from build123d import *

# Parameters (mm, degrees)
SKETCH1_W            = 350
SKETCH1_H            = 340
BOSS_EXTRUDE1_DEPTH  = 6
CUT_EXTRUDE2_DEPTH   = 6
MIRROR2_COPY_1_DEPTH = 6
CUT_EXTRUDE3_DEPTH   = 6
SKETCH4_W            = 10
SKETCH4_H            = 82.256980738
CUT_EXTRUDE4_DEPTH   = 6
SKETCH5_R            = 2.25
SKETCH5_R_2          = 1.75
CUT_EXTRUDE5_DEPTH   = 6
SKETCH6_W            = 12
SKETCH6_H            = 9
CUT_EXTRUDE6_DEPTH   = 6
SKETCH8_W            = 5
SKETCH8_H            = 3
CUT_EXTRUDE7_DEPTH   = 6
LPATTERN1_COUNT      = 3
LPATTERN1_PITCH      = 50
SKETCH9_W            = 3
SKETCH9_H            = 5
CUT_EXTRUDE8_DEPTH   = 6
LPATTERN2_COUNT      = 4
LPATTERN2_PITCH      = 50
SKETCH10_W           = 30
SKETCH10_H           = 25
CUT_EXTRUDE9_DEPTH   = 6
SKETCH11_W           = 10
SKETCH11_H           = 51.49656536
CUT_EXTRUDE10_DEPTH  = 6
SKETCH12_W           = 45
SKETCH12_H           = 45
CUT_EXTRUDE11_DEPTH  = 6
FILLET2_R            = 4.9
SKETCH13_R           = 2.75
CUT_EXTRUDE12_DEPTH  = 6
SKETCH14_W           = 50
SKETCH14_H           = 20
SKETCH14_W_2         = 40
CUT_EXTRUDE13_DEPTH  = 10
FILLET4_R            = 5
FILLET5_R            = 5
SKETCH15_W           = 65
SKETCH15_H           = 46.515736948
CUT_EXTRUDE14_DEPTH  = 10
FILLET6_R            = 10


with BuildPart() as part:
    # Sketch1 → Boss-Extrude1 (new body)
    with BuildSketch(Plane(origin=(0, 0, 0), x_dir=(1, 0, 0), z_dir=(0, 1, 0))):
        Rectangle(SKETCH1_W, SKETCH1_H)
    extrude(amount=BOSS_EXTRUDE1_DEPTH)

    # Sketch2 → Cut-Extrude2 (cut)
    with BuildSketch(Plane(origin=(0, 6, 0), x_dir=(1, 0, 0), z_dir=(0, 1, 0))):
        Polygon((-175, -130), (-155, -130), (-155, -150), (-135, -150), (-135, -170), (-175, -170), align=None)
    cut_extrude2 = extrude(amount=-CUT_EXTRUDE2_DEPTH, mode=Mode.SUBTRACT)

    # Mirror1: Cut-Extrude2 across plane
    add(cut_extrude2.mirror(Plane.XY), mode=Mode.SUBTRACT)

    # Mirror2: Cut-Extrude2 across plane
    add(cut_extrude2.mirror(Plane(origin=(0, 0, 0), x_dir=(0, 0, 1), z_dir=(1, 0, 0))), mode=Mode.SUBTRACT)

    # Mirror2 copy 1 sketch → Mirror2 copy 1 (cut)
    with BuildSketch(Plane(origin=(0, 6, 0), x_dir=(-1, 0, 0), z_dir=(0, 1, 0))):
        Polygon((-175, -130), (-155, -130), (-155, -150), (-135, -150), (-135, -170), (-175, -170), align=None)
    extrude(amount=-MIRROR2_COPY_1_DEPTH, mode=Mode.SUBTRACT)

    # Sketch3 → Cut-Extrude3 (cut)
    with BuildSketch(Plane(origin=(0, 6, 0), x_dir=(1, 0, 0), z_dir=(0, 1, 0))):
        Polygon((-22.5, 170), (-22.5, 150), (-11.5, 112), (11.5, 112), (22.5, 150), (22.5, 170), align=None)
    extrude(amount=-CUT_EXTRUDE3_DEPTH, mode=Mode.SUBTRACT)

    # Sketch4 → Cut-Extrude4 (cut)
    with BuildSketch(Plane(origin=(0, 6, 0), x_dir=(1, 0, 0), z_dir=(0, 1, 0))):
        with Locations((-97.5, 165.128490369)):
            Rectangle(SKETCH4_W, SKETCH4_H)
        with Locations((97.5, 165.128490369)):
            Rectangle(SKETCH4_W, SKETCH4_H)
    extrude(amount=-CUT_EXTRUDE4_DEPTH, mode=Mode.SUBTRACT)

    # Sketch5 → Cut-Extrude5 (cut)
    with BuildSketch(Plane(origin=(0, 6, 0), x_dir=(1, 0, 0), z_dir=(0, 1, 0))):
        with Locations(Location((104, 51.5, 0), (0, 0, 270))):
            Circle(SKETCH5_R)
        with Locations(Location((104, -99, 0), (0, 0, 270))):
            Circle(SKETCH5_R)
        with Locations(Location((54, -99, 0), (0, 0, 270))):
            Circle(SKETCH5_R)
        with Locations(Location((54, 51.5, 0), (0, 0, 270))):
            Circle(SKETCH5_R)
        with Locations(Location((-4.5, 33.75, 0), (0, 0, 270))):
            Circle(SKETCH5_R_2)
        with Locations(Location((-4.5, -81.25, 0), (0, 0, 270))):
            Circle(SKETCH5_R_2)
        with Locations(Location((-96.5, -81.25, 0), (0, 0, 270))):
            Circle(SKETCH5_R_2)
        with Locations(Location((-96.5, 33.75, 0), (0, 0, 270))):
            Circle(SKETCH5_R_2)
    extrude(amount=-CUT_EXTRUDE5_DEPTH, mode=Mode.SUBTRACT)

    # Sketch6 → Cut-Extrude6 (cut)
    with BuildSketch(Plane(origin=(0, 6, 0), x_dir=(1, 0, 0), z_dir=(0, 1, 0))):
        with Locations((-97.5, 145.5)):
            Rectangle(SKETCH6_W, SKETCH6_H)
        with Locations((97.5, 145.5)):
            Rectangle(SKETCH6_W, SKETCH6_H)
    extrude(amount=-CUT_EXTRUDE6_DEPTH, mode=Mode.SUBTRACT)

    # Sketch8 → Cut-Extrude7 (cut)
    with BuildSketch(Plane(origin=(0, 6, 0), x_dir=(1, 0, 0), z_dir=(0, 1, 0))):
        with Locations((-4.5, -125)):
            Rectangle(SKETCH8_W, SKETCH8_H)
        with Locations((-4.5, -145)):
            Rectangle(SKETCH8_W, SKETCH8_H)
    cut_extrude7 = extrude(amount=-CUT_EXTRUDE7_DEPTH, mode=Mode.SUBTRACT)

    # LPattern1: Cut-Extrude7 ×3
    with Locations(*[(-i * LPATTERN1_PITCH, 0, 0) for i in range(1, LPATTERN1_COUNT)]):
        add(cut_extrude7, mode=Mode.SUBTRACT)

    # Sketch9 → Cut-Extrude8 (cut)
    with BuildSketch(Plane(origin=(0, 6, 0), x_dir=(1, 0, 0), z_dir=(0, 1, 0))):
        with Locations((-150, -81.25)):
            Rectangle(SKETCH9_W, SKETCH9_H)
        with Locations((-130, -81.25)):
            Rectangle(SKETCH9_W, SKETCH9_H)
    cut_extrude8 = extrude(amount=-CUT_EXTRUDE8_DEPTH, mode=Mode.SUBTRACT)

    # LPattern2: Cut-Extrude8 ×4
    with Locations(*[(0, 0, -i * LPATTERN2_PITCH) for i in range(1, LPATTERN2_COUNT)]):
        add(cut_extrude8, mode=Mode.SUBTRACT)

    # Sketch10 → Cut-Extrude9 (cut)
    with BuildSketch(Plane(origin=(0, 6, 0), x_dir=(1, 0, 0), z_dir=(0, 1, 0))):
        with Locations((140, -157.5)):
            Rectangle(SKETCH10_W, SKETCH10_H)
    cut_extrude9 = extrude(amount=-CUT_EXTRUDE9_DEPTH, mode=Mode.SUBTRACT)

    # Mirror3: Cut-Extrude9 across plane
    add(cut_extrude9.mirror(Plane(origin=(0, 0, 0), x_dir=(0, 0, 1), z_dir=(1, 0, 0))), mode=Mode.SUBTRACT)

    # Sketch11 → Cut-Extrude10 (cut)
    with BuildSketch(Plane(origin=(0, 6, 0), x_dir=(1, 0, 0), z_dir=(0, 1, 0))):
        with Locations((55, 165.74828268)):
            Rectangle(SKETCH11_W, SKETCH11_H)
    extrude(amount=-CUT_EXTRUDE10_DEPTH, mode=Mode.SUBTRACT)

    # Sketch12 → Cut-Extrude11 (cut)
    with BuildSketch(Plane(origin=(0, 6, 0), x_dir=(1, 0, 0), z_dir=(0, 1, 0))):
        with Locations((-152.5, 147.5)):
            Rectangle(SKETCH12_W, SKETCH12_H)
    extrude(amount=-CUT_EXTRUDE11_DEPTH, mode=Mode.SUBTRACT)

    # Fillet2
    fillet2_edges = [part.edges().sort_by_distance(p)[0] for p in [
        (125, 3, 145),
        (-125, 3, 145),
        (50, 3, -140),
        (60, 3, -140),
        (-130, 3, -125),
    ]]
    fillet(fillet2_edges, radius=FILLET2_R)

    # Sketch13 → Cut-Extrude12 (cut)
    with BuildSketch(Plane(origin=(0, 6, 0), x_dir=(1, 0, 0), z_dir=(0, 1, 0))):
        with Locations(Location((165, -120, 0), (0, 0, 270))):
            Circle(SKETCH13_R)
        with Locations(Location((165, 120, 0), (0, 0, 270))):
            Circle(SKETCH13_R)
        with Locations(Location((125, 160, 0), (0, 0, 270))):
            Circle(SKETCH13_R)
        with Locations(Location((-120, 160, 0), (0, 0, 270))):
            Circle(SKETCH13_R)
        with Locations(Location((-165, 115, 0), (0, 0, 270))):
            Circle(SKETCH13_R)
        with Locations(Location((-165, -120, 0), (0, 0, 270))):
            Circle(SKETCH13_R)
        with Locations(Location((-115, -160, 0), (0, 0, 270))):
            Circle(SKETCH13_R)
        with Locations(Location((115, -160, 0), (0, 0, 270))):
            Circle(SKETCH13_R)
    extrude(amount=-CUT_EXTRUDE12_DEPTH, mode=Mode.SUBTRACT)

    # Sketch14 → Cut-Extrude13 (cut)
    with BuildSketch(Plane(origin=(0, 6, 0), x_dir=(1, 0, 0), z_dir=(0, 1, 0))):
        with Locations((82.5, 160)):
            Rectangle(SKETCH14_W, SKETCH14_H)
        with Locations((-87.5, 160)):
            Rectangle(SKETCH14_W_2, SKETCH14_H)
    extrude(amount=-CUT_EXTRUDE13_DEPTH, mode=Mode.SUBTRACT)

    # Fillet4
    fillet4_edges = [part.edges().sort_by_distance(p)[0] for p in [
        (-102.5, 3, -124),
        (-92.5, 3, -124),
    ]]
    fillet(fillet4_edges, radius=FILLET4_R - 0.0001)  # a hair under: the kernel refuses the full size

    # Fillet5
    fillet5_edges = [part.edges().sort_by_distance(p)[0] for p in [
        (92.5, 3, -124),
        (102.5, 3, -124),
    ]]
    fillet(fillet5_edges, radius=FILLET5_R - 0.0001)  # a hair under: the kernel refuses the full size

    # Sketch15 → Cut-Extrude14 (cut)
    with BuildSketch(Plane(origin=(0, 0, 0), x_dir=(-1, 0, 0), z_dir=(0, -1, 0))):
        with Locations((77.5, 146.742131526)):
            Rectangle(SKETCH15_W, SKETCH15_H)
        with Locations((-82.5, 146.742131526)):
            Rectangle(SKETCH15_W, SKETCH15_H)
    extrude(amount=-CUT_EXTRUDE14_DEPTH, mode=Mode.SUBTRACT)

    # Fillet6
    fillet6_edges = [part.edges().sort_by_distance(p)[0] for p in [
        (-110, 3, -123.484263052),
        (-45, 3, -123.484263052),
        (50, 3, -123.484263052),
        (115, 3, -123.484263052),
    ]]
    fillet(fillet6_edges, radius=FILLET6_R)


solid = part.part
For this review, take the finished solid that the model builds, in its own axes (mm). A direction names the side the tool comes from. Round coordinates to 2 decimals unless told otherwise and drop trailing zeros. Write each loop counter-clockwise with the first axis right and the second up, starting at its lowest first coordinate (ties: lowest second). Pieces come first, ordered by that corner, then holes. Notation, with made-up numbers: (-32.5, -25.75) -> (5.5, -25.75) arc R23 cw to (5.5, -7.75) -> close; hole circle Ø5 at (46.25, -20). An arc over 180 degrees is marked (long way). Put each result on its own line as item: value.
Q1. Consider section B-B on y = 2.65. Give the number of separate pieces and of enclosed holes in the cut face, and give its area (3 significant figures).
Determined:
separate pieces: 1
enclosed holes: 30
area: 104,000 mm^2
Q2. The part is to be moulded in two halves that separate along X. For faces 3 (the cylindrical face through (-48.007, 3.042, -126.336)), 4 (the flat face through (-17, 3, -131)), 5 (the flat face through (-2, 6, -2)), say which applies: released by +X, released by -X, zero draft, split by the parting line, or undercut.
Determined:
face 3: undercut
face 4: undercut
face 5: zero draft
Q3. Machinability: for faces 1 (the cylindrical face through (52.852, 3.042, -126.491)), 2 (the flat face through (-2, 0, -2)), which of the approach directions +Z, -Z, +X, -X, +Y, -Y give a long, thin tool a straight path to every point of the face, cutting with its end or side? Answer none if there is none.
Determined:
face 1: -Z, +Y, -Y
face 2: +Z, -Z, +X, -X, -Y
Q4. Consider section A-A on x = -71.5. State the section outline as (y, z) points, and give its area (3 significant figures).
Determined:
outline: (0, -123.48) -> (6, -123.48) -> (6, 170) -> (0, 170) -> close
area: 1,760 mm^2
Q5. To check wall thickness, follow L1, parallel to X at y = 3.9, z = -51.5; L2, parallel to X at y = 3.6, z = 120; L3, parallel to Z at x = -165, y = 2.9. State the ranges of each line that lie inside material, in increasing order. Write a range as [from, to].
Determined:
L1: x = [-175, 51.75], [56.25, 101.75], [106.25, 175]
L2: x = [-175, -167.75], [-162.25, 162.25], [167.75, 175]
L3: z = [-125, -117.75], [-112.25, 117.25], [122.75, 130]
Q6. Clearance check with flat-ended pins moving along their axes: pin 1 Ø6.5 at (x, z) = (165, -120) entering from -Y; pin 2 Ø1 at (x, y) = (137, 1.5) entering from -Z; pin 3 Ø1.8 at (y, z) = (3.5, -144.5) entering from +X; pin 4 Ø0.9 at (x, y) = (-130.5, 3) entering from +Z. State where each tip first meets the part, or that it passes through.
Determined:
pin 1: stops at y = 0
pin 2: stops at z = -150
pin 3: stops at x = 155
pin 4: stops at z = 145
